from build123d import *

# Parameters (mm, degrees)
SKETCH1_W           = 56.896
SKETCH1_H           = 27.94
BOSS_EXTRUDE1_DEPTH = 2.54
CUT_EXTRUDE1_DEPTH  = 3.54
FILLET1_R           = 1.27


with BuildPart() as part:
    # Sketch1 → Boss-Extrude1 (new body)
    with BuildSketch(Plane.XY):
        Rectangle(SKETCH1_W, SKETCH1_H)
    extrude(amount=BOSS_EXTRUDE1_DEPTH)

    # Sketch2 → Cut-Extrude1 (cut, through all)
    with BuildSketch(Plane.XY.offset(2.54)):
        with BuildLine():
            Line((-15.875, -13.97), (15.875, -13.97))
            ThreePointArc((15.875, -13.97), (0, -4.197045335), (-15.875, -13.97))
        make_face()
    extrude(amount=-CUT_EXTRUDE1_DEPTH, mode=Mode.SUBTRACT)

    # Fillet1
    fillet1_edges = [part.edges().sort_by_distance(p)[0] for p in [
        (-15.875, -13.97, 1.27),
        (15.875, -13.97, 1.27),
        (28.448, -13.97, 1.27),
        (-28.448, -13.97, 1.27),
        (-28.448, 13.97, 1.27),
        (28.448, 13.97, 1.27),
    ]]
    fillet(fillet1_edges, radius=FILLET1_R)


solid = part.part
Build history of the part. All positions in model axes, mm. A direction names the side the tool comes from. Coordinates: 2 decimals unless noted, no trailing zeros. Write each loop counter-clockwise with the first axis right and the second up, starting at its lowest first coordinate (ties: lowest second). Pieces come first, ordered by that corner, then holes.
(1) Pin check, flat tip, straight feed: pin 1 Ø4 at (x, y) = (5.5, -6.5) entering from -Z. Stop position of the tip, or through.
(2) Cut at A-A on y = -10.75. List the corners of the cut face in (x, z).
(3) 3-axis set-ups, long thin cutter, end or side, ignore diameter. For faces 4 (the cylindrical face through (16, -13.8, 1.3)), 5 (the flat face through (0, 13.97, 1)): which of +Z, -Z, +X, -X, +Y, -Y reach the whole face in a straight line?
(4) Cut at D-D on x = 3. List the corners of the cut face in (y, z).
(5) Cut at C-C on x = 10.5. List the corners of the cut face in (y, z).
(6) Mould opens along X. For faces 1 (the cylindrical face through (-16, -13.8, 1.3)), 2 (the cylindrical face through (-28.086, -13.588, 1.288)), 3 (the cylindrical face through (28.066, 13.608, 1.288)) say: pulls with the +X half, pulls with the -X half, needs draft (parallel to the pull), parting line crosses it, or undercut.
(7) Drill centre lines: line 1 (X direction, y = -9, z = 0.4); line 2 (Y direction, x = 16, z = 2.45); line 3 (Y direction, x = -6, z = 0.4). Where is each one in solid material? Low to high.
(8) Cut at B-B on z = 1.7. List the corners of the cut face in (x, y), and give its area (3 significant figures).
Working result:
1. pin 1: stops at z = 0
2. outline: (-28.45, 0) - (-13.79, 0) - (-13.79, 2.54) - (-28.45, 2.54) - close; (13.79, 0) - (28.45, 0) - (28.45, 2.54) - (13.79, 2.54) - close
3. face 4: +Z, -Z, -Y
3. face 5: +Z, -Z, +X, -X, +Y
4. outline: (-4.45, 0) - (13.97, 0) - (13.97, 2.54) - (-4.45, 2.54) - close
5. outline: (-7.63, 0) - (13.97, 0) - (13.97, 2.54) - (-7.63, 2.54) - close
6. face 1: undercut
6. face 2: pulls with the -X half
6. face 3: pulls with the +X half
7. line 1: x = -28.45 to -12.15, 12.15 to 28.45
7. line 2: y = -13.8 to 13.97
7. line 3: y = -5.24 to 13.97
8. outline: (-28.45, -12.7) arc R1.27 ccw to (-27.18, -13.97) - (-16.64, -13.97) arc R1.27 ccw to (-15.53, -13.32) arc R17.78 cw to (15.53, -13.32) arc R1.27 ccw to (16.64, -13.97) - (27.18, -13.97) arc R1.27 ccw to (28.45, -12.7) - (28.45, 12.7) arc R1.27 ccw to (27.18, 13.97) - (-27.18, 13.97) arc R1.27 ccw to (-28.45, 12.7) - close
8. area: 1,370 mm2
